The model under review builds one solid part; all positions refer to its coordinate system, in mm. Round coordinates to 2 decimals unless told otherwise and drop trailing zeros. Write each loop counter-clockwise with the first axis right and the second up, starting at its lowest first coordinate (ties: lowest second). Pieces come first, ordered by that corner, then holes. Notation, with made-up numbers: (37, 58) -> (48, 58) arc R13 cw to (48, 66) -> close; hole circle Ø7 at (-34.75, -15). An arc over 180 degrees is marked (long way). Answer in a Markdown table with one row per item. Add a question column.
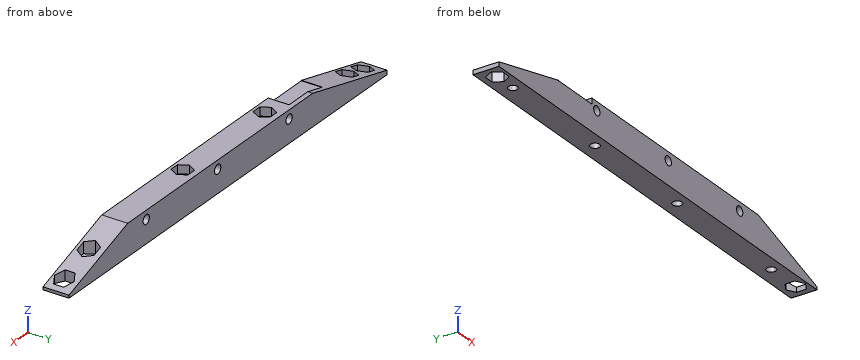
Autodesk Inventor part; units mm, degrees
ref_plane "YZ Plane" through (0, 0, 0) normal (1, 0, 0) x (0, 1, 0)
ref_plane "XZ Plane" through (0, 0, 0) normal (0, 1, 0) x (-1, 0, 0)
ref_plane "XY Plane" through (0, 0, 0) normal (0, 0, 1) x (1, 0, 0)
sketch "Sketch1" plane through (0, 0, 0) normal (0, 0, 1) x (1, 0, 0)
  line L0 (0, 0) -> (164.5, 0)
  line L1 (164.5, 0) -> (164.5, 9)
  line L2 (164.5, 9) -> (0, 9)
  line L3 (0, 9) -> (0, 0)
  circle A0 centre (57, 4) radius 1.6
  circle A1 centre (99, 4) radius 1.6
  circle A2 centre (159.5, 4) radius 1.6
  circle A3 centre (147, 4) radius 1.6
  circle A4 centre (15, 4) radius 1.6
  circle A5 centre (7, 4) radius 1.6
  dimension "d1" = 9
  dimension "d2" = 90
  dimension "d4" = 3.2
  dimension "d6" = 3.2
  dimension "d7" = 3.2
  dimension "d8" = 42
  dimension "d9" = 60.5
  dimension "d26" = 3.2
  dimension "d27" = 48
  dimension "d28" = 3.2
  dimension "d29" = 42
  dimension "d32" = 15
  dimension "d33" = 5
  dimension "d61" = 3.2
  dimension "d62" = 8
  dimension "d63" = 12.5
  dimension "d108" = 4
  dimension "d109" = 4
  dimension "d110" = 4
  dimension "d111" = 4
  dimension "d112" = 4
  dimension "d113" = 4
ref_plane "Work Plane2" through (0, 0, 0) normal (0, -1, 0) x (1, 0, 0)
sketch "Sketch2" plane through (0, 0, 0) normal (0, -1, 0) x (1, 0, 0)
  circle A0 centre (52, 8) radius 1.6
  circle A1 centre (125, 8) radius 1.6
  circle A2 centre (88.5, 8) radius 1.6
  point P0 (0, 0)
  point P1 (52, 0)
  dimension "d13" = 3.2
  dimension "d15" = 3.2
  dimension "d17" = 3.2
  dimension "d18" = 36.5
  dimension "d64" = 52
  dimension "d65" = 36.5
  dimension "d114" = 8
  dimension "d115" = 73
ref_plane "Work Plane1" through (0, 0, 11) normal (0, 0, 1) x (1, 0, 0)
extrude "klocek" add sketch "Sketch1" along normal blind 11
ref_plane "Work Plane3" through (0, 0, 0) normal (0, -1, 0) x (1, 0, 0)
extrude "prowadzenie osi" cut sketch "Sketch2" against normal up to next
ref_plane "Work Plane4" through (0, 0, 0) normal (0, -1, 0) x (1, 0, 0)
sketch "Sketch7" plane through (0, 0, 0) normal (0, -1, 0) x (1, 0, 0)
  line L0 (0, 11) -> (0, 1)
  line L1 (0, 11) -> (164.5, 11)
  line L2 (0, 11) -> (40, 11)
  line L3 (40, 11) -> (0, 1)
  point P0 (0, -1.8333)
  dimension "d86" = 10
  dimension "d87" = 40
sketch "Sketch8" plane through (0, 0, 0) normal (0, -1, 0) x (1, 0, 0)
  line L0 (164.5, 0) -> (164.5, 11)
  line L1 (164.5, 11) -> (164.5, 1)
  line L2 (164.5, 11) -> (0, 11)
  line L3 (164.5, 11) -> (134.5, 11)
  line L4 (134.5, 11) -> (164.5, 1)
  point P0 (0, 0)
  point P1 (40.8333, 11)
  dimension "d80" = 10
  dimension "d81" = 30
extrude "przedni skos" cut sketch "Sketch7" against normal up to next
extrude "tylni skos" cut sketch "Sketch8" against normal up to next
ref_plane "Work Plane7" through (0, 0, 11) normal (0, 0, 1) x (1, 0, 0)
sketch "Sketch5" plane through (0, 0, 11) normal (0, 0, 1) x (1, 0, 0)
  circle A0 centre (99, 4) radius 1.6
  line L0 (95.5936, 4) -> (97.2968, 6.95)
  line L1 (97.2968, 6.95) -> (100.7032, 6.95)
  line L2 (100.7032, 6.95) -> (102.4064, 4)
  line L3 (102.4064, 4) -> (100.7032, 1.05)
  line L4 (100.7032, 1.05) -> (97.2968, 1.05)
  line L5 (97.2968, 1.05) -> (95.5936, 4)
  circle A1 centre (57, 4) radius 1.6
  line L6 (60.4064, 4) -> (58.7032, 1.05)
  line L7 (58.7032, 1.05) -> (55.2968, 1.05)
  line L8 (55.2968, 1.05) -> (53.5936, 4)
  line L9 (53.5936, 4) -> (55.2968, 6.95)
  line L10 (55.2968, 6.95) -> (58.7032, 6.95)
  line L11 (58.7032, 6.95) -> (60.4064, 4)
  point P0 (119.5, 5)
  dimension "d98" = 5.9
  dimension "d100" = 5.9
extrude "hex insert middle" cut sketch "Sketch5" against normal blind 3
ref_plane "Work Plane6" through (0, 0, 11) normal (0, 0, 1) x (1, 0, 0)
sketch "Sketch9" plane through (0, 0, 11) normal (0, 0, 1) x (1, 0, 0)
  circle A0 centre (147, 4) radius 1.6
  line L0 (150.4064, 4) -> (148.7032, 1.05)
  line L1 (148.7032, 1.05) -> (145.2968, 1.05)
  line L2 (145.2968, 1.05) -> (143.5936, 4)
  line L3 (143.5936, 4) -> (145.2968, 6.95)
  line L4 (145.2968, 6.95) -> (148.7032, 6.95)
  line L5 (148.7032, 6.95) -> (150.4064, 4)
  point P0 (0, 0)
  point P1 (153, 5)
  dimension "d99" = 5.9
extrude "hex insert rear 1" cut sketch "Sketch9" against normal blind 7.5
ref_plane "Work Plane5" through (0, 0, 11) normal (0, 0, 1) x (1, 0, 0)
sketch "Sketch10" plane through (0, 0, 11) normal (0, 0, 1) x (1, 0, 0)
  circle A0 centre (159.5, 4) radius 1.6
  line L0 (162.45, 5.7032) -> (162.45, 2.2968)
  line L1 (162.45, 2.2968) -> (159.5, 0.5936)
  line L2 (159.5, 0.5936) -> (156.55, 2.2968)
  line L3 (156.55, 2.2968) -> (156.55, 5.7032)
  line L4 (156.55, 5.7032) -> (159.5, 7.4064)
  line L5 (159.5, 7.4064) -> (162.45, 5.7032)
  line L6 (164.5, 0) -> (134.5, 0)
  point P0 (0, 0)
  dimension "d118" = 5.9
extrude "hex insert rear 2" cut sketch "Sketch10" against normal up to next contours A0 | L0 L1 L2 L3 L4 L5
sketch "Sketch13" plane through (0, 0, 11) normal (0, 0, 1) x (1, 0, 0)
  circle A0 centre (7, 4) radius 1.6
  line L0 (10.4064, 4) -> (8.7032, 1.05)
  line L1 (8.7032, 1.05) -> (5.2968, 1.05)
  line L2 (5.2968, 1.05) -> (3.5936, 4)
  line L3 (3.5936, 4) -> (5.2968, 6.95)
  line L4 (5.2968, 6.95) -> (8.7032, 6.95)
  line L5 (8.7032, 6.95) -> (10.4064, 4)
  dimension "d123" = 5.9
extrude "hex insert front 1" cut sketch "Sketch13" against normal through all
sketch "Sketch16" plane through (0, 0, 11) normal (0, 0, 1) x (1, 0, 0)
  circle A0 centre (15, 4) radius 1.6
  line L0 (18.4064, 4) -> (16.7032, 1.05)
  line L1 (16.7032, 1.05) -> (13.2968, 1.05)
  line L2 (13.2968, 1.05) -> (11.5936, 4)
  line L3 (11.5936, 4) -> (13.2968, 6.95)
  line L4 (13.2968, 6.95) -> (16.7032, 6.95)
  line L5 (16.7032, 6.95) -> (18.4064, 4)
  point P0 (0, 0)
  dimension "d93" = 5.9
extrude "hex insert front 2" cut sketch "Sketch16" against normal blind 9
sketch "Sketch17" plane through (0, 0, 0) normal (0, 0, -1) x (-1, 0, 0)
  line L0 (-164.5, 9) -> (0, 9)
  line L1 (0, 0) -> (-2, 0)
  line L2 (-2, 0) -> (-2, 9)
  line L3 (-2, 9) -> (0, 9)
  line L4 (0, 9) -> (0, 0)
  dimension "d122" = 2
extrude "ciecie przod" cut sketch "Sketch17" against normal up to next
sketch "Sketch18" plane through (40, 0, 11) normal (0, -1, 0) x (1, 0, 0)
  line L0 (9.5, 0) -> (9.5, -2)
  line L1 (9.5, -2) -> (-7.5, -2)
  line L2 (-7.5, -2) -> (-7.5, 0)
  line L3 (-7.5, 0) -> (9.5, 0)
  line L4 (94.5, 0) -> (0, 0)
  circle A0 centre (12, -3) radius 1.6
  line L5 (-40, -11) -> (124.5, -11)
  point P0 (-35, -11)
  dimension "d102" = 2
  dimension "d103" = 17
  dimension "d104" = 2.5
extrude "sensor linii" cut sketch "Sketch18" against normal blind 7.3 contours L0 L1 L2 L3
properties part number "wheel_support_v4_narrow_with_line_sensor_all_holes"
1. Add section B-B on x = 15. Write out the cut boundary in (y, z), plus the area to 3 significant figures.
2. For L1, parallel to Z at x = 125, y = 4.75; L2, parallel to Y at x = 99, z = 3.25; L3, parallel to Z at x = 37, y = 1.25, list the stretches that pass through material, from the lowest coordinate up.
3. Add section A-A on x = 99. Write out the cut boundary in (y, z).
4. Insertion check: pin 1 Ø1.9 at (x, z) = (88.5, 8) entering from -Y; pin 2 Ø5 at (y, z) = (5.5, 5.5) entering from +X; pin 3 Ø3 at (x, y) = (56.5, 4.5) entering from +Z. Each pin has a flat end and moves straight along its axis. Give the tip position at first contact, or say it passes through.
Filled in:
| question | item | result |
|---|---|---|
| 1 | outline | (0, 0) -> (2.4, 0) -> (2.4, 2) -> (1.05, 2) -> (1.05, 4.75) -> (0, 4.75) -> close; (5.6, 0) -> (9, 0) -> (9, 4.75) -> (6.95, 4.75) -> (6.95, 2) -> (5.6, 2) -> close |
| 1 | area | 20.1 mm² |
| 2 | L1 | 0 to 6.4, 9.6 to 11 |
| 2 | L2 | 0 to 2.4, 5.6 to 9 |
| 2 | L3 | 0 to 9 |
| 3 | outline | (0, 0) -> (2.4, 0) -> (2.4, 8) -> (1.05, 8) -> (1.05, 11) -> (0, 11) -> close; (5.6, 0) -> (9, 0) -> (9, 11) -> (6.95, 11) -> (6.95, 8) -> (5.6, 8) -> close |
| 4 | pin 1 | through |
| 4 | pin 2 | x = 157.9 |
| 4 | pin 3 | z = 8 |
